CAD build for the part. Positions are in the model's coordinates, mm. Give positions to 0.01 mm unless a question says otherwise; leave off trailing zeros. Answer as a JSON object with one key per item and string values.
Autodesk Inventor part; units mm, degrees
ref_plane "YZ Plane" through (0, 0, 0) normal (1, 0, 0) x (0, 1, 0)
ref_plane "XZ Plane" through (0, 0, 0) normal (0, 1, 0) x (-1, 0, 0)
ref_plane "XY Plane" through (0, 0, 0) normal (0, 0, 1) x (1, 0, 0)
sketch "Skizze1" plane through (0, 0, 0) normal (0, 0, 1) x (1, 0, 0)
  line L0 (-397.5, 166.5) -> (397.5, 166.5)
  line L1 (397.5, 166.5) -> (397.5, -166.5)
  line L2 (397.5, -166.5) -> (-397.5, -166.5)
  line L3 (-397.5, -166.5) -> (-397.5, 166.5)
  line L4 (-397.5, 166.5) -> (397.5, -166.5) construction
  line L5 (397.5, 166.5) -> (-397.5, -166.5) construction
  line L6 (-357.5, 126.5) -> (357.5, 126.5)
  line L7 (357.5, 126.5) -> (357.5, -126.5)
  line L8 (357.5, -126.5) -> (-357.5, -126.5)
  line L9 (-357.5, -126.5) -> (-357.5, 126.5)
  line L10 (0, 233.1) -> (0, -233.1) construction
  line L11 (-397.5, 46.5) -> (-357.5, 46.5)
  line L12 (-357.5, 46.5) -> (-277.5, 126.5)
  line L13 (-277.5, 126.5) -> (-277.5, 166.5)
  line L14 (-397.5, -46.5) -> (-357.5, -46.5)
  line L15 (-357.5, -46.5) -> (-277.5, -126.5)
  line L16 (-277.5, -126.5) -> (-277.5, -166.5)
  line L17 (357.5, 46.5) -> (277.5, 126.5)
  line L18 (277.5, 126.5) -> (277.5, 166.5)
  line L19 (397.5, -46.5) -> (357.5, -46.5)
  line L20 (357.5, -46.5) -> (277.5, -126.5)
  line L21 (392.5, 161.5) -> (-392.5, 161.5)
  line L22 (-392.5, 161.5) -> (-392.5, -161.5)
  line L23 (-392.5, -161.5) -> (392.5, -161.5)
  line L24 (392.5, -161.5) -> (392.5, 161.5)
  circle A0 centre (-207.5, -60) radius 2.75
  line L25 (-556.5, 0) -> (556.5, 0) construction
  circle A1 centre (-207.5, 60) radius 2.75
  circle A2 centre (207.5, -60) radius 2.75
  circle A3 centre (207.5, 60) radius 2.75
  line L26 (-385.5, -45) -> (-369.5, -45) construction
  line L27 (-369.5, -45) -> (-369.5, 45) construction
  line L28 (-369.5, 45) -> (-385.5, 45) construction
  line L29 (-385.5, 45) -> (-385.5, -45) construction
  line L30 (-385.5, -45) -> (-369.5, 45) construction
  line L31 (-369.5, -45) -> (-385.5, 45) construction
  circle A4 centre (-377.5, -7.5) radius 3.25
  circle A5 centre (-377.5, -37) radius 4.5
  line L32 (-369.5, 0) -> (-385.5, 0) construction
  line L33 (-377.5, -45) -> (-377.5, 45) construction
  circle A6 centre (-377.5, 37) radius 4.5
  circle A7 centre (-377.5, 7.5) radius 3.25
  line L34 (-47.5, 154.5) -> (47.5, 154.5) construction
  line L35 (47.5, 154.5) -> (47.5, 138.5) construction
  line L36 (47.5, 138.5) -> (-47.5, 138.5) construction
  line L37 (-47.5, 138.5) -> (-47.5, 154.5) construction
  line L38 (-47.5, 154.5) -> (47.5, 138.5) construction
  line L39 (47.5, 154.5) -> (-47.5, 138.5) construction
  line L40 (-47.5, 146.5) -> (47.5, 146.5) construction
  circle A8 centre (-7.5, 146.5) radius 3.25
  circle A9 centre (-37, 146.5) radius 4.5
  circle A10 centre (7.5, 146.5) radius 3.25
  circle A11 centre (37, 146.5) radius 4.5
  circle A12 centre (377.5, -37) radius 4.5
  circle A13 centre (377.5, -7.5) radius 3.25
  circle A14 centre (377.5, 7.5) radius 3.25
  circle A15 centre (377.5, 37) radius 4.5
  circle A16 centre (0, 0) radius 2.5
  circle A17 centre (80, 0) radius 2.5
  circle A18 centre (160, 0) radius 2.5
  circle A19 centre (240, 0) radius 2.5
  circle A20 centre (320, 0) radius 2.5
  circle A21 centre (-80, 0) radius 2.5
  circle A22 centre (-160, 0) radius 2.5
  circle A23 centre (-240, 0) radius 2.5
  circle A24 centre (-320, 0) radius 2.5
  line L41 (-282.5, -121.5) -> (282.5, -121.5)
  line L42 (397.5, 46.5) -> (357.5, 46.5)
  line L43 (277.5, -126.5) -> (277.5, -166.5)
  point P0 (0, 0)
  point P1 (277.5, 161.5)
  point P2 (-277.5, 161.5)
  point P3 (-392.5, 46.5)
  point P4 (-392.5, -46.5)
  point P5 (-310.6574, -126.5)
  point P6 (277.5, -126.5)
  point P7 (392.5, -46.5)
  point P8 (-207.5, 0)
  point P9 (-377.5, 0)
  point P10 (0, 146.5)
  point P11 (392.5, 46.5)
  point P12 (277.5, -161.5)
  point P13 (-277.5, -161.5)
  dimension "d0" = 795
  dimension "d1" = 333
  dimension "d2" = 40
  dimension "d13" = 5
  dimension "d16" = 5.5
  dimension "d22" = 60
  dimension "d25" = 16
  dimension "d26" = 90
  dimension "d27" = 6.5
  dimension "d28" = 9
  dimension "d29" = 7.5
  dimension "d30" = 37
  dimension "d33" = 20
  dimension "d34" = 95
  dimension "d35" = 16
  dimension "d36" = 20
  dimension "d37" = 6.5
  dimension "d38" = 9
  dimension "d39" = 7.5
  dimension "d40" = 37
  dimension "d41" = 5
  dimension "d44" = 80
  dimension "d51" = 80
  dimension "d56" = 5
  dimension "d57" = 121.5
  dimension "d58" = 120
  dimension "d59" = 120
  dimension "d60" = 120
  dimension "d61" = 120
extrude "Extrusion1" add sketch "Skizze1" along normal blind 3 contours L21 L18 L6 L13 | L11 L9 L14 L22 | L6 L17 L7 L20 L41 L15 L9 L12 | L24 L19 L7 L42
chamfer "Fase-5mm" distance 5 angle 45 6 edges at (-277.5, 161.5, 1.5) (277.5, 161.5, 1.5) (392.5, 46.5, 1.5) (392.5, -46.5, 1.5) (-392.5, -46.5, 1.5) (-392.5, 46.5, 1.5)
equation "\"d37\" = d27"
equation "\"d38\" = d28"
equation "\"d39\" = d29"
equation "\"d40\" = d30"
equation "\"d59\" = d58"
equation "\"d60\" = d58"
equation "\"d61\" = d58"
properties part number "enc - SidePanel Oben V2"
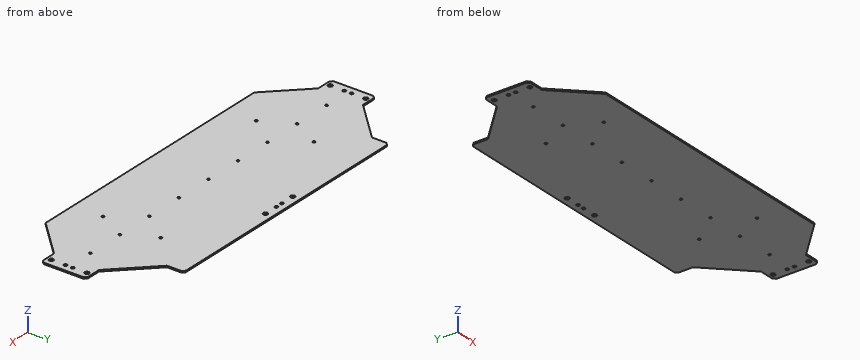
1) Slice it at A-A (z = 0.55). State how many separate pieces and enclosed holes the cut face has, then the cut area to 3 significant figures.
Model answer:
{"separate pieces": "1", "enclosed holes": "25", "area": "190,000 mm2"}
2) Wall check: probe 1 along Y at (x, z) = (-207.5, 1.8); probe 2 along Y at (x, z) = (80, 2.2); probe 3 along Y at (x, z) = (-37, 1.4). Give the ranges that are in metal, low to high.
Model answer:
{"probe 1": "y = -121.5 to -62.75, -57.25 to 57.25, 62.75 to 161.5", "probe 2": "y = -121.5 to -2.5, 2.5 to 161.5", "probe 3": "y = -121.5 to 142, 151 to 161.5"}
3) Pin check, flat tips, straight feed: pin 1 (8.5 mm diameter, centred on x = 7.5, y = 146.5, fed in from -Z); pin 2 (0.9 mm diameter, centred on y = 146.5, z = 1, fed in from -X); pin 3 (7 mm diameter, centred on x = 377.5, y = 37, fed in from -Z); pin 4 (1 mm diameter, centred on y = 126.5, z = 1.5, fed in from -X). Stop position of each tip, or through.
Model answer:
{"pin 1": "stops at z = 0", "pin 2": "stops at x = -277.5", "pin 3": "passes through", "pin 4": "stops at x = -278"}
